```python
from build123d import *

# Parameters (mm, degrees)
SKETCH1_W           = 30
SKETCH1_H           = 30
BOSS_EXTRUDE1_DEPTH = 10


with BuildPart() as part:
    # Sketch1 → Boss-Extrude1 (new, symmetric)
    with BuildSketch(Plane(origin=(0, 0, 0), x_dir=(1, 0, 0), z_dir=(0, 1, 0))):
        with BuildLine():
            Line((-20, 30), (20, 30))
            ThreePointArc((20, 30), (27.071067812, 27.071067812), (30, 20))
            Line((30, 20), (30, -20))
            ThreePointArc((30, -20), (27.071067812, -27.071067812), (20, -30))
            Line((20, -30), (-20, -30))
            ThreePointArc((-20, -30), (-27.071067812, -27.071067812), (-30, -20))
            Line((-30, -20), (-30, 20))
            ThreePointArc((-30, 20), (-27.071067812, 27.071067812), (-20, 30))
        make_face()
        Rectangle(SKETCH1_W, SKETCH1_H, mode=Mode.SUBTRACT)
    extrude(amount=BOSS_EXTRUDE1_DEPTH, both=True)


solid = part.part
```
Work out the finished part from the listing and answer in its coordinate system (mm). A direction names the side the tool comes from. Round coordinates to 2 decimals unless told otherwise and drop trailing zeros. Order: outer loops, then holes, each group sorted by start corner. A loop starts at its lowest first (then second) coordinate and runs counter-clockwise, first axis right, second up.
Q1. A cutting plane is placed at A-A, the plane z = 5.5. Determine the outline of the cut face in (x, y), then the cut area to 3 significant figures.
Solution:
outline: (-30, -10) - (-15, -10) - (-15, 10) - (-30, 10) - close; (15, -10) - (30, -10) - (30, 10) - (15, 10) - close
area: 600 mm2
Q2. A cutting plane is placed at B-B, the plane y = -3. Determine the outline of the cut face in (x, z).
Solution:
outline: (-30, -20) arc R10 ccw to (-20, -30) - (20, -30) arc R10 ccw to (30, -20) - (30, 20) arc R10 ccw to (20, 30) - (-20, 30) arc R10 ccw to (-30, 20) - close; hole (-15, -15) - (15, -15) - (15, 15) - (-15, 15) - close
Q3. A cutting plane is placed at C-C, the plane x = 2.5. Determine the outline of the cut face in (y, z).
Solution:
outline: (-10, -30) - (10, -30) - (10, -15) - (-10, -15) - close; (-10, 15) - (10, 15) - (10, 30) - (-10, 30) - close
Q4. Find the intervals of material crossed by line 1 along X through (y, z) = (2, -11.5); line 2 along X through (y, z) = (-6.75, 21), in increasing order.
Solution:
line 1: x = -30 to -15, 15 to 30
line 2: x = -29.95 to 29.95
Q5. A cutting plane is placed at D-D, the plane x = -26. Determine the outline of the cut face in (y, z), then the cut area to 3 significant figures.
Solution:
outline: (-10, -28) - (10, -28) - (10, 28) - (-10, 28) - close
area: 1,120 mm2
Q6. A tool of negligible diameter and unlimited length cuts with its end or side. For faces 1 (the flat face through (0, 0, -15)), 2 (the flat face through (0, -10, 20)), from which of +Z, -Z, +X, -X, +Y, -Y can it reach the whole face along a straight path? Write none if from no direction.
Solution:
face 1: +Y, -Y
face 2: +Z, -Z, +X, -X, -Y
Q7. The mould has two halves that part along X. Classify faces 3 (the cylindrical face through (-27.15, 0.14, -26.99)), 4 (the flat face through (0, 0, 30)), 5 (the flat face through (0, 0, 15)): pulls with the +X half, pulls with the -X half, needs draft (parallel to the pull), parting line crosses it, or undercut.
Solution:
face 3: pulls with the -X half
face 4: needs draft
face 5: undercut
